```python
from build123d import *

# Parameters (mm, degrees)
SKETCH_1_W          = 60
SKETCH_1_H          = 12
CUT_EXTRUDE_2_DEPTH = 23


with BuildPart() as part:
    # Эскиз1 → Повернуть1 (revolve)
    with BuildSketch(Plane.XY, mode=Mode.PRIVATE) as revolve_1_sk:
        with Locations((30, 6)):
            Rectangle(SKETCH_1_W, SKETCH_1_H)
    revolve(revolve_1_sk.sketch.rotate(Axis((0, 0, 0), (1, 0, 0)), 90), axis=Axis((0, 0, 0), (1, 0, 0)))

    # Эскиз2 → Вырез-Вытянуть2 (cut, symmetric)
    with BuildSketch(Plane.ZY.offset(-30)):
        Polygon((3, 77.578035125), (3, 11.618950039), (3, -11.618950039), (3, -77.578035125), (134.918170173, -77.578035125), (134.918170173, 77.578035125), align=None)
    cut_extrude_2 = extrude(amount=CUT_EXTRUDE_2_DEPTH, both=True, mode=Mode.SUBTRACT)

    # Зеркальное отражение1: Вырез-Вытянуть2 across plane
    add(cut_extrude_2.mirror(Plane.XY), mode=Mode.SUBTRACT)


solid = part.part
```
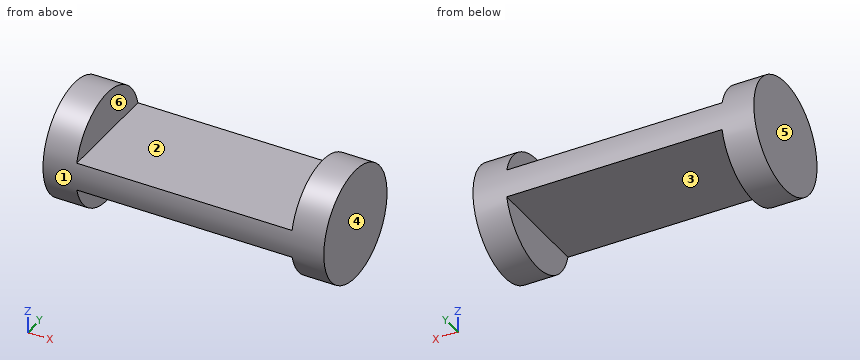
Geometry: final body of the model. Coordinates: model frame, mm. Face numbers are marked on the shaded views. A direction names the side the tool comes from. Give positions to 0.01 mm unless a question says otherwise; leave off trailing zeros. Write each loop counter-clockwise with the first axis right and the second up, starting at its lowest first coordinate (ties: lowest second). Pieces come first, ordered by that corner, then holes.
1. Reachability of the marked faces 1, 2 and 3 from +Z, -Z, +X, -X, +Y, -Y: full face, straight path, thin tool, end or side. Return the list, or none.
2. Line query: probe 1 along X at (y, z) = (-9, 6.75); probe 2 along Z at (x, y) = (38.5, -3); probe 3 along Y at (x, z) = (21, -0.25). Output: solid intervals per line, ascending.
3. Section query B-B, the plane y = 3. Return loops of the section in (x, z), then the cut area to 3 significant figures.
4. Section query C-C, the plane x = 36. Return loops of the section in (y, z).
5. Section query A-A, the plane z = -8.25. Return loops of the section in (x, y), then the cut area to 3 significant figures.
6. Draft query along X for the marked faces 4, 5 and 6. Return one class per face: released by +X, released by -X, zero draft, split by the parting line, or undercut.
7. Pin query (flat end, axial travel): P1, Ø8, axis at x = 15, y = 2.5, coming from the +Z side; P2, Ø6, axis at x = 30, z = 3.5, coming from the -Y side; P3, Ø10, axis at x = 35, y = 2, coming from the -Z side. Return the tip coordinate at first contact, or that it passes through.
8. Section query D-D, the plane z = 5.5. Return loops of the section in (x, y), then the cut area to 3 significant figures.
Computed:
1. face 1: +X, -X
1. face 2: +Z, +Y, -Y
1. face 3: -Z, +Y, -Y
2. probe 1: x = 0 to 7, 53 to 60
2. probe 2: z = -3 to 3
2. probe 3: y = -12 to 12
3. outline: (0, -11.62) - (7, -11.62) - (7, -3) - (53, -3) - (53, -11.62) - (60, -11.62) - (60, 11.62) - (53, 11.62) - (53, 3) - (7, 3) - (7, 11.62) - (0, 11.62) - close
3. area: 601 mm2
4. outline: (-11.62, -3) - (11.62, -3) arc R12 ccw to (11.62, 3) - (-11.62, 3) arc R12 ccw to start
5. outline: (0, -8.71) - (7, -8.71) - (7, 8.71) - (0, 8.71) - close; (53, -8.71) - (60, -8.71) - (60, 8.71) - (53, 8.71) - close
5. area: 244 mm2
6. face 4: released by +X
6. face 5: released by -X
6. face 6: undercut
7. P1: stops at z = 3
7. P2: stops at y = -11.99
7. P3: stops at z = -3
8. outline: (0, -10.67) - (7, -10.67) - (7, 10.67) - (0, 10.67) - close; (53, -10.67) - (60, -10.67) - (60, 10.67) - (53, 10.67) - close
8. area: 299 mm2
